Verification items for the finished model (mm, model axes). A direction names the side the tool comes from. Round coordinates to 2 decimals unless told otherwise and drop trailing zeros. Write each loop counter-clockwise with the first axis right and the second up, starting at its lowest first coordinate (ties: lowest second). Pieces come first, ordered by that corner, then holes. Notation, with made-up numbers: (25.25, -16.75) - (76.25, -16.75) arc R5 cw to (76.25, -11.75) - close; hole circle Ø2 at (-5.75, -11.5). An arc over 180 degrees is marked (long way). Answer as a JSON object with one key per item and string values.
```python
from build123d import *

# Parameters (mm, degrees)
BOSS_EXTRUDE1_DEPTH = 6.35


with BuildPart() as part:
    # Sketch1 → Boss-Extrude1 (new body)
    with BuildSketch(Plane.XY):
        Polygon((0, -6.35), (19.05, -6.35), (19.05, 0), (24.15, 0), (24.15, 3.175), (22.15, 3.175), (22.15, 5.175), (24.15, 5.175), (24.15, 9.525), (26.65, 9.525), (26.65, 5.175), (28.65, 5.175), (28.65, 3.175), (26.65, 3.175), (26.65, 0), (34.925, 0), (41.275, 0), (41.275, 10.795), (34.925, 10.795), (34.925, 19.07), (31.115, 19.07), (31.115, 17.07), (29.115, 17.07), (29.115, 19.07), (24.765, 19.07), (24.765, 21.57), (29.115, 21.57), (29.115, 23.57), (31.115, 23.57), (31.115, 21.57), (34.925, 21.57), (34.925, 29.845), (41.275, 29.845), (41.275, 60.325), (34.925, 60.325), (26.65, 60.325), (26.65, 56.515), (28.65, 56.515), (28.65, 54.515), (26.65, 54.515), (26.65, 50.165), (24.15, 50.165), (24.15, 54.515), (22.15, 54.515), (22.15, 56.515), (24.15, 56.515), (24.15, 60.325), (19.05, 60.325), (19.05, 66.675), (0, 66.675), (0, 60.325), (-5.1, 60.325), (-5.1, 56.515), (-3.1, 56.515), (-3.1, 54.515), (-5.1, 54.515), (-5.1, 50.165), (-7.6, 50.165), (-7.6, 54.515), (-9.6, 54.515), (-9.6, 56.515), (-7.6, 56.515), (-7.6, 60.325), (-15.875, 60.325), (-22.225, 60.325), (-22.225, 29.845), (-15.875, 29.845), (-15.875, 21.57), (-12.065, 21.57), (-12.065, 23.57), (-10.065, 23.57), (-10.065, 21.57), (-5.715, 21.57), (-5.715, 19.07), (-10.065, 19.07), (-10.065, 17.07), (-12.065, 17.07), (-12.065, 19.07), (-15.875, 19.07), (-15.875, 10.795), (-22.225, 10.795), (-22.225, 0), (-15.875, 0), (-7.6, 0), (-7.6, 3.175), (-9.6, 3.175), (-9.6, 5.175), (-7.6, 5.175), (-7.6, 9.525), (-5.1, 9.525), (-5.1, 5.175), (-3.1, 5.175), (-3.1, 3.175), (-5.1, 3.175), (-5.1, 0), (0, 0), align=None)
    extrude(amount=BOSS_EXTRUDE1_DEPTH)


solid = part.part
```
Q1. Material ranges on line 1 along X through (y, z) = (17.5, 2.25) (3 decimals); line 2 along X through (y, z) = (4, 3) (3 decimals); line 3 along Y through (x, z) = (-16.5, 3.5) (3 decimals), recorded low to high. Write a range as [from, to].
Geometry check:
{"line 1": "x = [-15.875, -12.065], [-10.065, 29.115], [31.115, 34.925]", "line 2": "x = [-22.225, -9.6], [-3.1, 22.15], [28.65, 41.275]", "line 3": "y = [0, 10.795], [29.845, 60.325]"}
Q2. Set-up check for faces 1 (the flat face through (25, 9.525, 3)), 2 (the flat face through (22, 60.325, 3)), 3 (the flat face through (23, 3.175, 3)), 4 (the flat face through (-3, 60.325, 3)): record each of +Z, -Z, +X, -X, +Y, -Y from which the full face is reachable in a straight line by a thin tool's end or side.
Geometry check:
{"face 1": "+Z, -Z, -Y", "face 2": "+Z, -Z, +X, +Y", "face 3": "+Z, -Z", "face 4": "+Z, -Z, -X, +Y"}
Q3. Section check C-C, the plane x = 20.5. Record the cut outline in (y, z) (3 decimals), then the cut area to 3 significant figures.
Geometry check:
{"outline": "(0, 0) - (60.325, 0) - (60.325, 6.35) - (0, 6.35) - close", "area": "383 mm2"}
Q4. Section check B-B, the plane x = 36.5. Record the cut outline in (y, z) (3 decimals), then the cut area to 3 significant figures.
Geometry check:
{"outline": "(0, 0) - (10.795, 0) - (10.795, 6.35) - (0, 6.35) - close; (29.845, 0) - (60.325, 0) - (60.325, 6.35) - (29.845, 6.35) - close", "area": "262 mm2"}
Q5. Section check A-A, the plane y = 6.5. Record the cut outline in (x, z) (3 decimals).
Geometry check:
{"outline": "(-22.225, 0) - (-7.6, 0) - (-7.6, 6.35) - (-22.225, 6.35) - close; (-5.1, 0) - (24.15, 0) - (24.15, 6.35) - (-5.1, 6.35) - close; (26.65, 0) - (41.275, 0) - (41.275, 6.35) - (26.65, 6.35) - close"}
Q6. Release check for a two-part mould opening along X. For faces 5 (the flat face through (-10.065, 23, 3)), 6 (the flat face through (27, 21.57, 3)), 7 (the flat face through (0, -3, 3)) record: released by +X, released by -X, zero draft, split by the parting line, or undercut.
Geometry check:
{"face 5": "undercut", "face 6": "zero draft", "face 7": "released by -X"}
Q7. Gauge pin test, flat ends, axial feed: P1, Ø0.6, axis at y = 22.5, z = 4.5, coming from the +X side (3 decimals); P2, Ø2, axis at y = 23, z = 4.5, coming from the -X side (3 decimals); P3, Ø3, axis at x = 30.5, z = 2, coming from the -Y side. Record the tip position at first contact, or that the pin passes through.
Geometry check:
{"P1": "stops at x = 34.925", "P2": "stops at x = -15.875", "P3": "stops at y = 0"}
